Geometry check sheet. Reference: the model listing, model coordinates, mm. Give positions to 0.01 mm unless a question says otherwise; leave off trailing zeros.
from build123d import *

# Parameters (mm, degrees)
SKETCH1_W           = 558.8
SKETCH1_H           = 25.4
BOSS_EXTRUDE1_DEPTH = 3.175
SKETCH2_R           = 2.413
CUT_EXTRUDE1_DEPTH  = 280.706508013
SKETCH3_R           = 3.302
CUT_EXTRUDE2_DEPTH  = 280.706508013


with BuildPart() as part:
    # Sketch1 → Boss-Extrude1 (new body)
    with BuildSketch(Plane(origin=(0, 0, 0), x_dir=(1, 0, 0), z_dir=(0, 1, 0))):
        Rectangle(SKETCH1_W, SKETCH1_H)
    extrude(amount=BOSS_EXTRUDE1_DEPTH)

    # Sketch2 → Cut-Extrude1 (cut, through all)
    with BuildSketch(Plane(origin=(0, 3.175, 0), x_dir=(1, 0, 0), z_dir=(0, 1, 0))):
        with Locations(Location((-266.7, 0, 0), (0, 0, 270))):
            Circle(SKETCH2_R)
        with Locations(Location((-241.3, 0, 0), (0, 0, 270))):
            Circle(SKETCH2_R)
        with Locations(Location((-215.9, 0, 0), (0, 0, 270))):
            Circle(SKETCH2_R)
    extrude(amount=-CUT_EXTRUDE1_DEPTH, mode=Mode.SUBTRACT)

    # Sketch3 → Cut-Extrude2 (cut, through all)
    with BuildSketch(Plane(origin=(0, 3.175, 0), x_dir=(1, 0, 0), z_dir=(0, 1, 0))):
        with Locations(Location((-152.4, 0, 0), (0, 0, 270))):
            Circle(SKETCH3_R)
        with Locations(Location((-127, 0, 0), (0, 0, 270))):
            Circle(SKETCH3_R)
        with Locations(Location((-12.7, 0, 0), (0, 0, 270))):
            Circle(SKETCH3_R)
        with Locations(Location((12.7, 0, 0), (0, 0, 270))):
            Circle(SKETCH3_R)
        with Locations(Location((127, 0, 0), (0, 0, 270))):
            Circle(SKETCH3_R)
        with Locations(Location((152.4, 0, 0), (0, 0, 270))):
            Circle(SKETCH3_R)
    extrude(amount=-CUT_EXTRUDE2_DEPTH, mode=Mode.SUBTRACT)


solid = part.part
Item 1: Gauge pin test, flat end, axial feed: pin 1 (6 mm diameter, centred on x = 127, z = 0, fed in from -Y). Record the tip position at first contact, or that the pin passes through.
Reported:
pin 1: passes through
Item 2: Scan lines: L1, parallel to Z at x = -266.7, y = 0.95; L2, parallel to Z at x = -126, y = 1.45. Record each from-to range of solid material in increasing order.
Reported:
L1: z = -12.7 to -2.41, 2.41 to 12.7
L2: z = -12.7 to -3.15, 3.15 to 12.7
Item 3: Sectioned sample at A-A (y = 1.3). Give the number of separate pieces and of enclosed holes in the cut face, and give its area (3 significant figures).
Reported:
separate pieces: 1
enclosed holes: 9
area: 13,900 mm2
